Source: CAD feature listing. Evaluate the final solid. Frame: model axes, mm. Face numbers are marked on the shaded views. Round coordinates to 2 decimals unless told otherwise and drop trailing zeros. Loops run counter-clockwise (first coordinate to the right, second up) from the corner with the lowest first, then second, coordinate; pieces in that order, holes last. Notation, with made-up numbers: (-5, 84) -> (24, 84) arc R14 cw to (24, 93) -> close; hole circle Ø7 at (-11, 82). An arc over 180 degrees is marked (long way). Put each result on its own line as item: value. Start each with the question number.
1. Material intervals for L1, parallel to Z at x = 31.5, y = 10; L2, parallel to Y at x = 34.5, z = 58.5; L3, parallel to X at y = 12, z = 25, sorted ascending.
2. Cut plane B-B (x = 7.5). Return the cut outline in (y, z), then the cut area to 3 significant figures.
3. Draft query along X for the marked faces 1, 2 and 3. Return one class per face: pulls with the +X half, pulls with the -X half, needs draft (parallel to the pull), parting line crosses it, or undercut.
4. Cut plane A-A (y = 32). Return the cut outline in (x, z).
5. Contact query for flat-ended pins moving along their axis: pin 1 (8 mm diameter, centred on x = 12, z = 14, fed in from -Y); pin 2 (3 mm diameter, centred on x = 17, z = 37, fed in from -Y); pin 3 (16.5 mm diameter, centred on x = 20, y = 14.5, fed in from +Z). Output: stop coordinate, or through.
6. Cut plane C-C (z = 51). Return the cut outline in (x, y).
```python
from build123d import *

# Parameters (mm, degrees)
F0_W     = 40
F0_H     = 40
F1_DEPTH = 70
F2_R     = 16.6382118991
F3_DEPTH = 80
F4_W     = 40
F4_H     = 40
F5_DEPTH = 8
F6_R     = 7


with BuildPart() as f1:
    # F0 (on Top) → F1 (new body)
    with BuildSketch(Plane.XY):
        with Locations((20, 20)):
            Rectangle(F0_W, F0_H)
    extrude(amount=F1_DEPTH)

    # F2 (on Top) → F3 (cut)
    with BuildSketch(Plane.XY):
        with Locations((19.8019631207, 19.8019631207)):
            Circle(F2_R)
    extrude(amount=F3_DEPTH, mode=Mode.SUBTRACT)

    # F4 (on Top) → F5 (join)
    with BuildSketch(Plane.XY):
        with Locations((20, 20)):
            Rectangle(F4_W, F4_H)
    extrude(amount=F5_DEPTH)

    # F8: sweep along a path in F7
    with BuildLine(Plane.YZ) as f8_path:
        Line((-5.8375704102, 26.8986206502), (5.3797238506, 19.1151890904))
    # F6 (on Front) → F8 (sweep, cut)
    with BuildSketch(Plane.XZ):
        with Locations((18.6525676399, 32.8138060868)):
            Circle(F6_R)
    sweep(path=f8_path.line, mode=Mode.SUBTRACT)


solid = f1.part
```
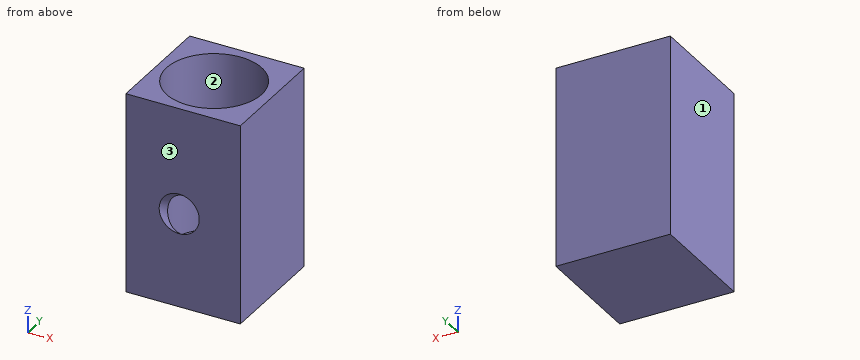
Solution:
1. L1: z = 0 to 8
1. L2: y = 0 to 12, 27.6 to 40
1. L3: x = 0 to 5.11, 34.5 to 40
2. outline: (0, 0) -> (40, 0) -> (40, 70) -> (31, 70) -> (31, 8) -> (8.6, 8) -> (8.6, 70) -> (0, 70) -> close
2. area: 1,410 mm^2
3. face 1: pulls with the -X half
3. face 2: undercut
3. face 3: needs draft
4. outline: (0, 0) -> (40, 0) -> (40, 70) -> (31.12, 70) -> (31.12, 8) -> (8.49, 8) -> (8.49, 70) -> (0, 70) -> close
5. pin 1: stops at y = 0
5. pin 2: stops at y = 1.53
5. pin 3: stops at z = 8
6. outline: (0, 0) -> (40, 0) -> (40, 40) -> (0, 40) -> close; hole circle Ø33.28 at (19.8, 19.8)
